Verification items for the finished model (mm, model axes). Face numbers are marked on the shaded views. A direction names the side the tool comes from. Round coordinates to 2 decimals unless told otherwise and drop trailing zeros. Order: outer loops, then holes, each group sorted by start corner. A loop starts at its lowest first (then second) coordinate and runs counter-clockwise, first axis right, second up. Notation, with made-up numbers: (85, -14) -> (108, -14) arc R28 ccw to (108, 5) -> close; hole circle Ø6 at (32, -20). An arc over 180 degrees is marked (long way). Answer in a Markdown table with one row per item. Add a question column.
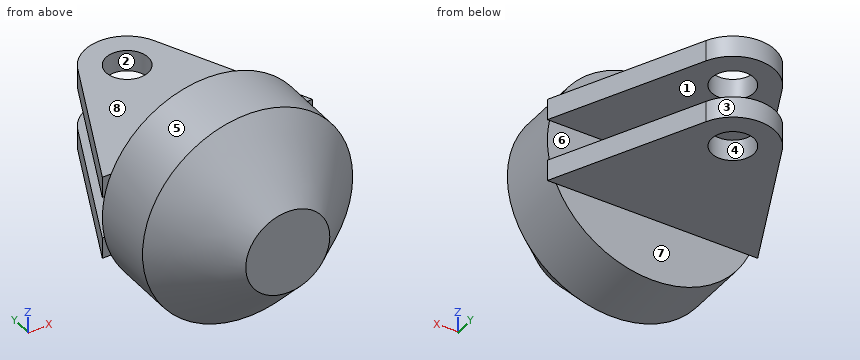
```python
from build123d import *

# Parameters (mm, degrees)
RESSALTO_EXTRUS_O1_START = 10
ESBO_O2_R                = 10
RESSALTO_EXTRUS_O1_DEPTH = 10


with BuildPart() as part:
    # Esboço1 → Revolução1 (revolve)
    with BuildSketch(Plane.XY):
        Polygon((0, 0), (0, 60), (50, 60), (50, 30), (20, 0), align=None)
    revolve(axis=Axis((0, 0, 0), (0, 1, 0)))

    # Esboço2 → Ressalto-extrusão1 (add)
    with BuildSketch(Plane.XY.offset(RESSALTO_EXTRUS_O1_START)):
        with BuildLine():
            Line((50, 60), (18.13082184, 128.442351533))
            ThreePointArc((18.13082184, 128.442351533), (0, 140), (-18.13082184, 128.442351533))
            Line((-18.13082184, 128.442351533), (-50, 60))
            Line((-50, 60), (50, 60))
        make_face()
        with Locations((0, 120)):
            Circle(ESBO_O2_R, mode=Mode.SUBTRACT)
    ressalto_extrus_o1 = extrude(amount=RESSALTO_EXTRUS_O1_DEPTH)

    # Espelhar1: Ressalto-extrusão1 across plane
    add(ressalto_extrus_o1.mirror(Plane.XY))


solid = part.part
```
1) Cross-section at C-C, the plane z = 0. Record the boundary of the cut face in (x, y).
2) Cross-section at B-B, the plane y = 93. Record the boundary of the cut face in (x, z), and give its area (3 significant figures).
3) Thickness scan on L1, parallel to Z at x = -25.5, y = 66.5; L2, parallel to X at y = 53.5, z = 32; L3, parallel to Y at x = -8.5, z = -5.5. Record the ranges inside material, lowest first. Write a range as [from, to].
4) Depth check by flat-ended pin: P1, Ø1.5, axis at y = 43, z = -36, coming from the +X side; P2, Ø10, axis at x = -31.5, z = 37, coming from the -Y side; P3, Ø4.5, axis at x = 48, z = -14, coming from the -Y side. Enter the tip coordinate at first touch or a pass-through.
5) Cross-section at D-D, the plane y = 120. Record the boundary of the cut face in (x, z).
6) Cross-section at A-A, the plane x = 0. Record the boundary of the cut face in (y, z), and give its area (3 significant figures).
7) Tool access check on the marked faces 5, 6, 7 and 8. Record the directions out of +Z, -Z, +X, -X, +Y, -Y that give a thin tool (end or side, any length) a straight path to the whole face; none if there is none.
8) Draft check along X on the marked faces 1, 2, 3 and 4. Enter one of: +X half, -X half, draft (parallel to the pull), parting line (faces both ways), or undercut.
Results below:
| question | item | result |
|---|---|---|
| 1 | outline | (-50, 30) -> (-20, 0) -> (20, 0) -> (50, 30) -> (50, 60) -> (-50, 60) -> close |
| 2 | outline | (-34.63, -20) -> (34.63, -20) -> (34.63, -10) -> (-34.63, -10) -> close; (-34.63, 10) -> (34.63, 10) -> (34.63, 20) -> (-34.63, 20) -> close |
| 2 | area | 1,390 mm² |
| 3 | L1 | [-20, -10], [10, 20] |
| 3 | L2 | [-38.42, 38.42] |
| 3 | L3 | [0, 60] |
| 4 | P1 | x = 35.46 |
| 4 | P2 | y = 23.59 |
| 4 | P3 | y = 27.75 |
| 5 | outline | (-22.06, -20) -> (-10, -20) -> (-10, -10) -> (-22.06, -10) -> close; (-22.06, 10) -> (-10, 10) -> (-10, 20) -> (-22.06, 20) -> close; (10, -20) -> (22.06, -20) -> (22.06, -10) -> (10, -10) -> close; (10, 10) -> (22.06, 10) -> (22.06, 20) -> (10, 20) -> close |
| 6 | outline | (0, -20) -> (30, -50) -> (60, -50) -> (60, -20) -> (110, -20) -> (110, -10) -> (60, -10) -> (60, 10) -> (110, 10) -> (110, 20) -> (60, 20) -> (60, 50) -> (30, 50) -> (0, 20) -> close; (130, -20) -> (140, -20) -> (140, -10) -> (130, -10) -> close; (130, 10) -> (140, 10) -> (140, 20) -> (130, 20) -> close |
| 6 | area | 6,300 mm² |
| 7 | face 5 | -Y |
| 7 | face 6 | +X, -X, +Y |
| 7 | face 7 | -Z, +X, -X, +Y |
| 7 | face 8 | +Z, +X, -X, +Y |
| 8 | face 1 | draft |
| 8 | face 2 | undercut |
| 8 | face 3 | parting line |
| 8 | face 4 | undercut |
